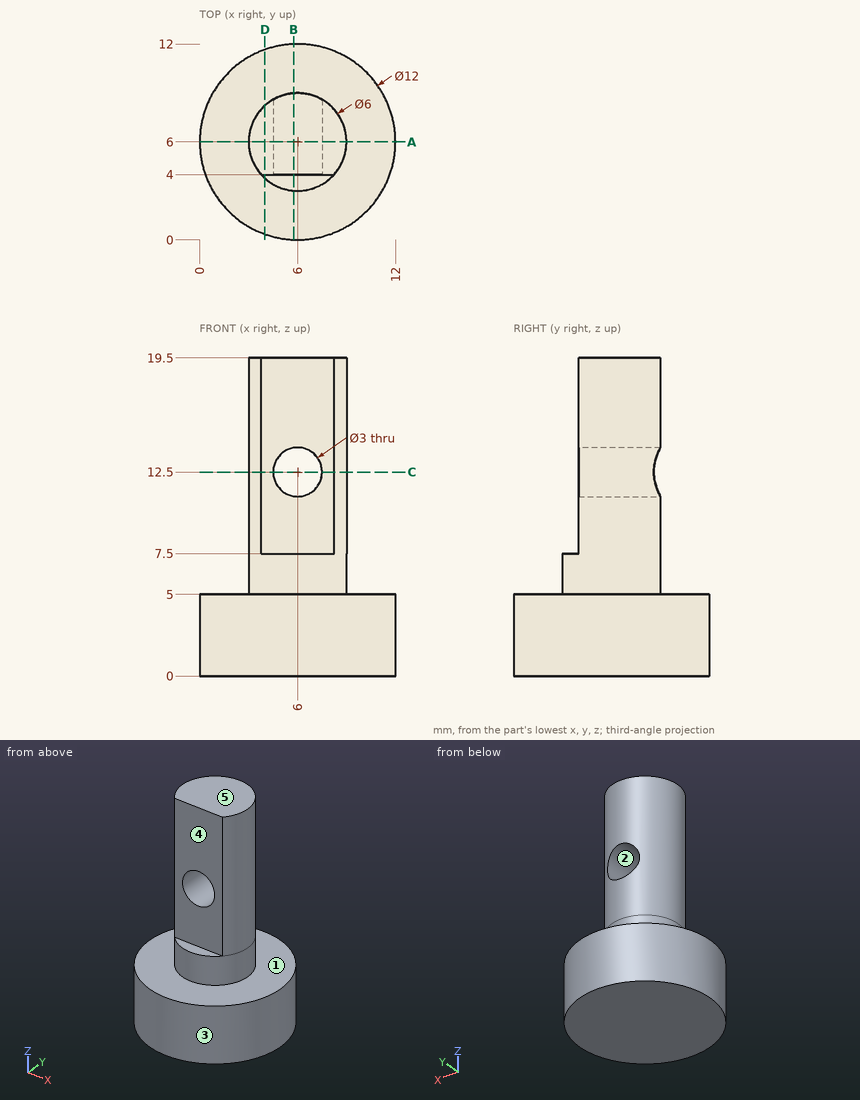
Print and shaded views of the part. All mm, measured from the part's lowest x, y and z. A direction names the side the tool comes from. Give positions to 0.01 mm unless a question says otherwise; leave off trailing zeros. Order: outer loops, then holes, each group sorted by start corner. A loop starts at its lowest first (then second) coordinate and runs counter-clockwise, first axis right, second up. Notation, with made-up numbers: (68, 57.5) - (109, 57.5) arc R15 ccw to (109, 62.5) - close; hole circle Ø11 at (34, 49.5). An arc over 180 degrees is marked (long way). One line per item, written item: value.
Item 1: Wall check: line 1 (Z direction, x = 6, y = 5.5); line 2 (X direction, y = 5.95, z = 12.5); line 3 (Z direction, x = 3, y = 10). Give the ranges that are in metal, low to high.
Response values:
line 1: 0 to 11, 14 to 19.5
line 2: 3 to 4.5, 7.5 to 9
line 3: 0 to 5
Item 2: Slice it at C-C (z = 12.5). List the corners of the cut face in (x, y), then the cut area to 3 significant figures.
Response values:
outline: (3.76, 4) - (4.5, 4) - (4.5, 8.6) arc R3 ccw to start; (7.5, 4) - (8.24, 4) arc R3 ccw to (7.5, 8.6) - close
area: 10.6 mm2
Item 3: Slice it at A-A (y = 6). List the corners of the cut face in (x, z).
Response values:
outline: (0, 0) - (12, 0) - (12, 5) - (9, 5) - (9, 19.5) - (3, 19.5) - (3, 5) - (0, 5) - close; hole circle Ø3 at (6, 12.5)
Item 4: Pin check, flat tips, straight feed: pin 1 Ø2 at (y, z) = (5.5, 13.5) entering from -X; pin 2 Ø4 at (x, z) = (6, 12.5) entering from +Y; pin 3 Ø3.5 at (x, z) = (5, 10.5) entering from -Y. Stop position of each tip, or through.
Response values:
pin 1: x = 3
pin 2: y = 9
pin 3: y = 4
Item 5: Slice it at B-B (x = 5.75). List the corners of the cut face in (y, z), then the cut area to 3 significant figures.
Response values:
outline: (0.01, 0) - (11.99, 0) - (11.99, 5) - (8.99, 5) - (8.99, 11.02) - (4, 11.02) - (4, 7.5) - (3.01, 7.5) - (3.01, 5) - (0.01, 5) - close; (4, 13.98) - (8.99, 13.98) - (8.99, 19.5) - (4, 19.5) - close
area: 120 mm2
Item 6: Tool access for the marked faces 4 and 5: list every direction of +Z, -Z, +X, -X, +Y, -Y with a clear straight run to the whole face (end or side of a thin tool).
Response values:
face 4: +Z, +X, -X, -Y
face 5: +Z, +X, -X, +Y, -Y
Item 7: Slice it at D-D (x = 4). List the corners of the cut face in (y, z), then the cut area to 3 significant figures.
Response values:
outline: (0.34, 0) - (11.66, 0) - (11.66, 5) - (8.24, 5) - (8.24, 19.5) - (4, 19.5) - (4, 7.5) - (3.76, 7.5) - (3.76, 5) - (0.34, 5) - close
area: 119 mm2
Item 8: Two-plate mould, pull along X, no slides. Class the marked faces 1, 2 and 3: released by +X, released by -X, zero draft, split by the parting line, or undercut.
Response values:
face 1: zero draft
face 2: undercut
face 3: split by the parting line
